Can you work these out from the model? Positions are in its coordinate system, mm. Face numbers are marked on the shaded views. Coordinates: 2 decimals unless noted, no trailing zeros. Order: outer loops, then holes, each group sorted by start corner. A loop starts at its lowest first (then second) coordinate and runs counter-clockwise, first axis right, second up.
```python
from build123d import *

# Parameters (mm, degrees)
SKETCH_1_R          = 15
SKETCH_1_R_2        = 10
EXTRUDE_1_DEPTH     = 6
CUT_EXTRUDE_1_REACH = 32
SKETCH_2_R          = 1.5
CUT_EXTRUDE_2_REACH = 37.49
SKETCH_3_R          = 1.5


with BuildPart() as part:
    # 스케치1 → 보스-돌출1 (new body)
    with BuildSketch(Plane(origin=(0, 0, 0), x_dir=(1, 0, 0), z_dir=(0, 1, 0))):
        Circle(SKETCH_1_R)
        Circle(SKETCH_1_R_2, mode=Mode.SUBTRACT)
    extrude(amount=EXTRUDE_1_DEPTH)

    # 스케치2 → 컷-돌출1 (cut, up to next)
    with BuildSketch(Plane(origin=(0, 0, -15), x_dir=(-1, 0, 0), z_dir=(0, 0, -1)), mode=Mode.PRIVATE) as cut_extrude_1_sk1:
        with Locations((0, 3)):
            Circle(SKETCH_2_R)
    cut_extrude_1_tool1 = extrude(cut_extrude_1_sk1.sketch, amount=-CUT_EXTRUDE_1_REACH, mode=Mode.PRIVATE) & part.part
    add(cut_extrude_1_tool1.solids().sort_by_distance((0, 3, -15))[0], mode=Mode.SUBTRACT)

    # 스케치3 → 컷-돌출2 (cut, up to next)
    with BuildSketch(Plane(origin=(-12.990381057, 0, 7.5), x_dir=(0, -1, 0), z_dir=(-0.866025404, 0, 0.5)), mode=Mode.PRIVATE) as cut_extrude_2_sk1:
        with Locations((-3, 0)):
            Circle(SKETCH_3_R)
    cut_extrude_2_tool1 = extrude(cut_extrude_2_sk1.sketch, amount=-CUT_EXTRUDE_2_REACH, mode=Mode.PRIVATE) & part.part
    add(cut_extrude_2_tool1.solids().sort_by_distance((-12.990381, 3, 7.5))[0], mode=Mode.SUBTRACT)


solid = part.part
```
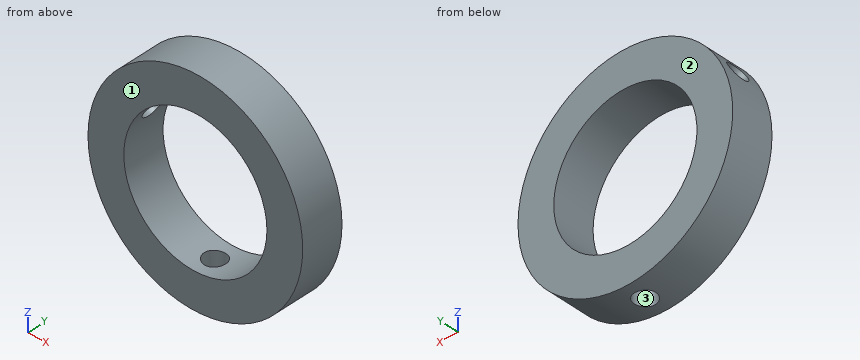
1. Imagine slicing it at B-B on x = 0. Please give me the cut outline in (y, z), then the cut area to 3 significant figures.
Completed:
outline: (0, -15) - (1.5, -15) - (1.5, -10) - (0, -10) - close; (0, 10) - (6, 10) - (6, 15) - (0, 15) - close; (4.5, -15) - (6, -15) - (6, -10) - (4.5, -10) - close
area: 45.0 mm2
2. Imagine slicing it at C-C on x = -4.5. Please give me the cut outline in (y, z).
Completed:
outline: (0, -14.31) - (6, -14.31) - (6, -8.93) - (0, -8.93) - close; (0, 8.93) - (6, 8.93) - (6, 14.31) - (0, 14.31) - close
3. Imagine slicing it at D-D on y = 1. Please give me the cut outline in (x, z), then the cut area to 3 significant figures.
Completed:
outline: circle Ø30 at (0, 0); hole circle Ø20 at (0, 0)
area: 393 mm2
4. Thinking about a two-plate mould opening in Y: for the marked faces 1, 2 and 3, which applies, pulls with the +Y half, pulls with the -Y half, needs draft (parallel to the pull), parting line crosses it, or undercut?
Completed:
face 1: pulls with the -Y half
face 2: pulls with the +Y half
face 3: undercut
5. Please list where these lines run through material, in increasing order: probe 1 along X at (y, z) = (3, 0); probe 2 along X at (y, z) = (3, -13.6).
Completed:
probe 1: x = -15 to -10, 10 to 15
probe 2: x = -6.33 to -1.5, 1.5 to 6.33
6. Imagine slicing it at A-A on z = 0. Please give me the cut outline in (x, y), then the cut area to 3 significant figures.
Completed:
outline: (-15, 0) - (-10, 0) - (-10, 6) - (-15, 6) - close; (10, 0) - (15, 0) - (15, 6) - (10, 6) - close
area: 60.0 mm2
7. I'm going to push flat-ended pins straight in: pin 1 (2.5 mm diameter, centred on x = 0, y = 3, fed in from -Z); pin 2 (2 mm diameter, centred on y = 3.5, z = -5, fed in from +X); pin 3 (1 mm diameter, centred on y = 2.5, z = 5.5, fed in from -X). Where does each tip first touch, or does it pass through?
Completed:
pin 1: stops at z = 9.92
pin 2: stops at x = 14.46
pin 3: stops at x = -14.14
